```python
from build123d import *

# Parameters (mm, degrees)
BOSS_EXTRUDE2_DEPTH = 5
SKETCH2_W           = 5
SKETCH2_H           = 30
CUT_EXTRUDE4_DEPTH  = 100
SKETCH3_R           = 11
CUT_EXTRUDE5_DEPTH  = 100
SKETCH5_W           = 45
SKETCH5_H           = 30
CUT_EXTRUDE6_DEPTH  = 100


with BuildPart() as part:
    # Sketch1 → Boss-Extrude2 (new body)
    with BuildSketch(Plane(origin=(0, 0, 0), x_dir=(1, 0, 0), z_dir=(0, 1, 0))):
        Polygon((70, -55), (15, -55), (15, -65), (-15, -65), (-15, -55), (-70, -55), (-70, 55), (-15, 55), (-15, 65), (15, 65), (15, 55), (70, 55), align=None)
    extrude(amount=BOSS_EXTRUDE2_DEPTH)

    # Sketch2 → Cut-Extrude4 (cut)
    with BuildSketch(Plane(origin=(0, 5, 0), x_dir=(1, 0, 0), z_dir=(0, 1, 0))):
        with Locations((-57.5, 0)):
            Rectangle(SKETCH2_W, SKETCH2_H)
        with Locations((57.5, 0)):
            Rectangle(SKETCH2_W, SKETCH2_H)
    extrude(amount=-CUT_EXTRUDE4_DEPTH, mode=Mode.SUBTRACT)

    # Sketch3 → Cut-Extrude5 (cut)
    with BuildSketch(Plane(origin=(0, 0, 0), x_dir=(-1, 0, 0), z_dir=(0, -1, 0))):
        with Locations(Location((0, 0, 0), (0, 0, 90))):
            Circle(SKETCH3_R)
    extrude(amount=-CUT_EXTRUDE5_DEPTH, mode=Mode.SUBTRACT)

    # Sketch5 → Cut-Extrude6 (cut)
    with BuildSketch(Plane(origin=(0, 0, 0), x_dir=(-1, 0, 0), z_dir=(0, -1, 0))):
        with Locations((47.5, -40)):
            Rectangle(SKETCH5_W, SKETCH5_H)
        with Locations((47.5, 40)):
            Rectangle(SKETCH5_W, SKETCH5_H)
        with Locations((-47.5, 40)):
            Rectangle(SKETCH5_W, SKETCH5_H)
        with Locations((-47.5, -40)):
            Rectangle(SKETCH5_W, SKETCH5_H)
    extrude(amount=-CUT_EXTRUDE6_DEPTH, mode=Mode.SUBTRACT)


solid = part.part
```
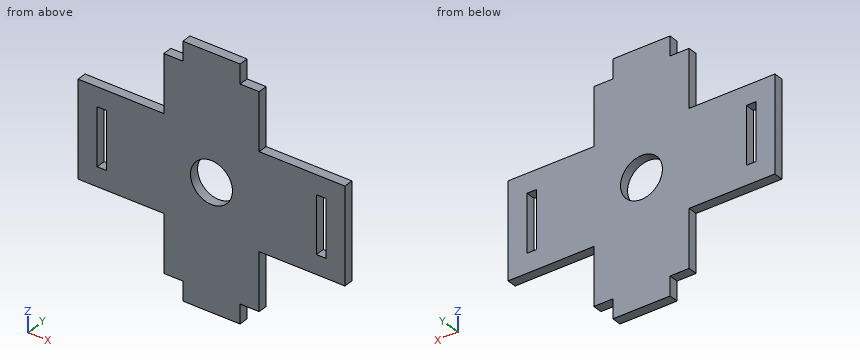
Work out the finished part from the listing and answer in its coordinate system (mm). Give positions to 0.01 mm unless a question says otherwise; leave off trailing zeros. Write each loop counter-clockwise with the first axis right and the second up, starting at its lowest first coordinate (ties: lowest second). Pieces come first, ordered by that corner, then holes.
(1) The part is cut by section D-D on z = -52.5. Write down the section's boundary in (x, y).
Final values:
outline: (-25, 0) - (25, 0) - (25, 5) - (-25, 5) - close
(2) Flat-ended cylindrical pins translate along their axes: pin 1 Ø2.5 at (x, y) = (22, 1.5) entering from -Z; pin 2 Ø1.5 at (y, z) = (3.5, 62.5) entering from +X; pin 3 Ø1 at (x, y) = (-32, 4.5) entering from -Z. Find the tip coordinate at first contact, or state that the pin passes through.
Final values:
pin 1: stops at z = -55
pin 2: stops at x = 15
pin 3: stops at z = -25
(3) The part is cut by section C-C on x = 0. Write down the section's boundary in (y, z), plus the area to 3 significant figures.
Final values:
outline: (0, -65) - (5, -65) - (5, -11) - (0, -11) - close; (0, 11) - (5, 11) - (5, 65) - (0, 65) - close
area: 540 mm2
(4) The part is cut by section A-A on z = 0. Write down the section's boundary in (x, y), plus the area to 3 significant figures.
Final values:
outline: (-70, 0) - (-60, 0) - (-60, 5) - (-70, 5) - close; (-55, 0) - (-11, 0) - (-11, 5) - (-55, 5) - close; (11, 0) - (55, 0) - (55, 5) - (11, 5) - close; (60, 0) - (70, 0) - (70, 5) - (60, 5) - close
area: 540 mm2
(5) Straight lines are drawn through the part: line 1 (X direction, y = 3.55, z = 0); line 2 (Z direction, x = 59, y = 3.55); line 3 (Z direction, x = 34.5, y = 3.95). For each, find the intervals that lie inside material, in ascending order.
Final values:
line 1: x = -70 to -60, -55 to -11, 11 to 55, 60 to 70
line 2: z = -25 to -15, 15 to 25
line 3: z = -25 to 25
(6) The part is cut by section B-B on y = 2.1. Count the separate pieces of the cut face and the enclosed holes in it, plus the area to 3 significant figures.
Final values:
separate pieces: 1
enclosed holes: 3
area: 9,920 mm2
